Verification items for this drawing (mm, ordinates from the low corner). Round coordinates to 2 decimals unless told otherwise and drop trailing zeros. Order: outer loops, then holes, each group sorted by start corner. A loop starts at its lowest first (then second) coordinate and runs counter-clockwise, first axis right, second up. Notation, with made-up numbers: M 49.25,34 L 85.25,34 A22 ccw 85.25,65 Z; hole C 26,25.25 d3. An arc over 180 degrees is marked long. One line per item, written item: value. Start each with the question number.
(1) Cross-section at A-A, the plane x = 163. Enter the section's corners in (y, z), and give its area (3 significant figures).
(2) Cross-section at C-C, the plane z = 1.8. Count the separate pieces of the cut face and the enclosed holes in it, and give its area (3 significant figures).
(3) Cross-section at D-D, the plane x = 206.5. Enter the section's corners in (y, z), and give its area (3 significant figures).
(4) Cross-section at B-B, the plane y = 30. Enter the section's corners in (x, z).
(5) Thickness scan on L1, parallel to X at y = 29.5, z = 2.9; L2, parallel to Y at x = 84.5, z = 1.05 (1 decimal); L3, parallel to Y at x = 82.5, z = 3.15. Record the ranges inside material, lowest first.
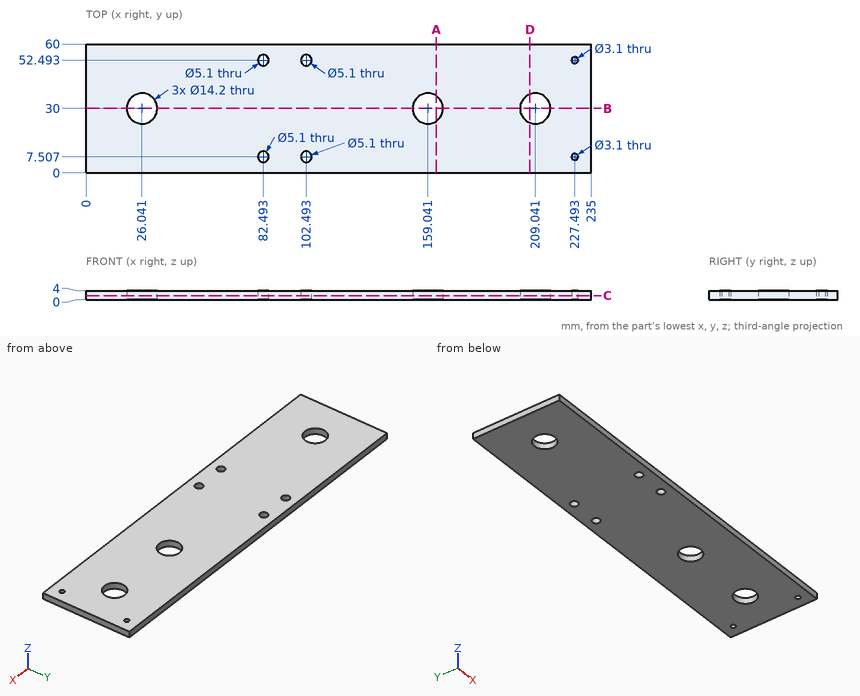
Values found:
1. outline: M 0,0 L 24.11,0 L 24.11,4 L 0,4 Z; M 35.89,0 L 60,0 L 60,4 L 35.89,4 Z
1. area: 193 mm^2
2. separate pieces: 1
2. enclosed holes: 9
2. area: 13,500 mm^2
3. outline: M 0,0 L 23.37,0 L 23.37,4 L 0,4 Z; M 36.63,0 L 60,0 L 60,4 L 36.63,4 Z
3. area: 187 mm^2
4. outline: M 0,0 L 18.94,0 L 18.94,4 L 0,4 Z; M 33.14,0 L 151.94,0 L 151.94,4 L 33.14,4 Z; M 166.14,0 L 201.94,0 L 201.94,4 L 166.14,4 Z; M 216.14,0 L 235,0 L 235,4 L 216.14,4 Z
5. L1: 0 to 18.96, 33.12 to 151.96, 166.12 to 201.96, 216.12 to 235
5. L2: 0 to 5.9, 9.1 to 50.9, 54.1 to 60
5. L3: 0 to 4.96, 10.06 to 49.94, 55.04 to 60
